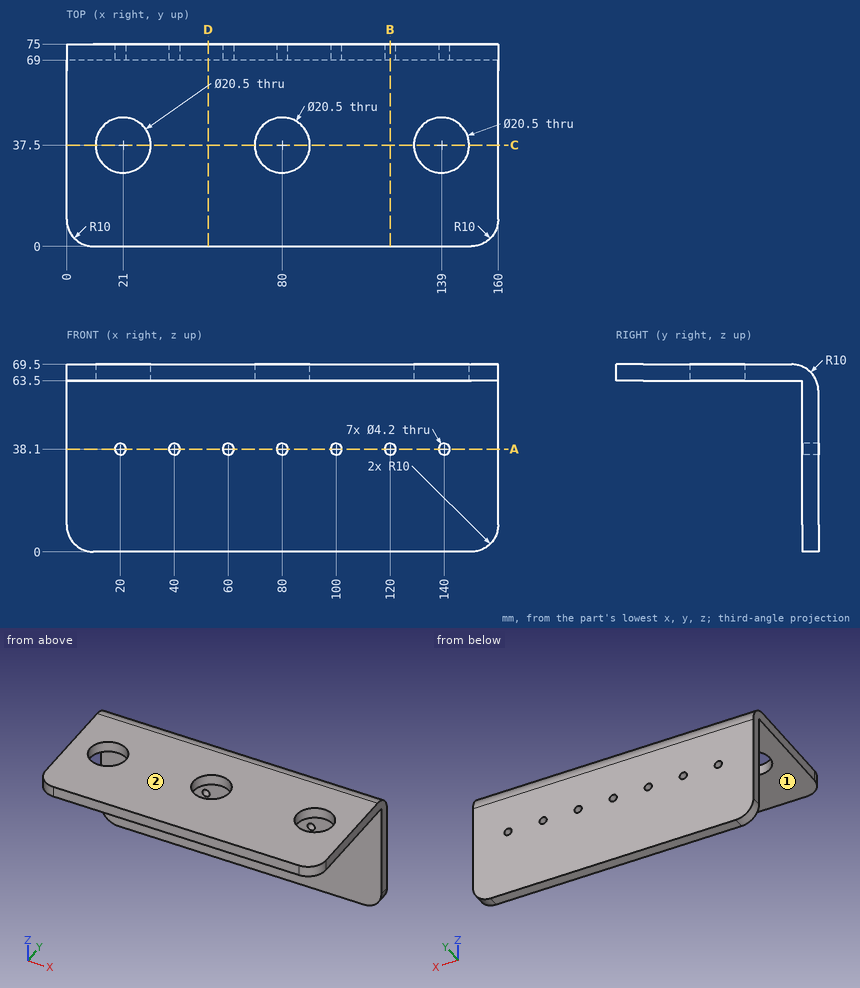
Part print with two shaded views. Sizes in mm from the minimum x, y, z corner. A direction names the side the tool comes from. Round coordinates to 2 decimals unless told otherwise and drop trailing zeros. Order: outer loops, then holes, each group sorted by start corner. A loop starts at its lowest first (then second) coordinate and runs counter-clockwise, first axis right, second up. Notation, with made-up numbers: (67.5, 42) - (104.5, 42) arc R32 cw to (104.5, 73) - close; hole circle Ø4 at (22.5, 56). An arc over 180 degrees is marked (long way). Answer in a Markdown table with one row per item. Add a question column.
(1) Drop flat-ended pins along their axis: pin 1 Ø3.5 at (x, z) = (100, 38.1) entering from +Y; pin 2 Ø12 at (x, z) = (106.5, 7.5) entering from -Y; pin 3 Ø23.5 at (x, y) = (21, 37.5) entering from -Z. Give the stop position or say it passes through.
(2) 3-axis set-ups, long thin cutter, end or side, ignore diameter. For the marked faces 1 and 2: which of +Z, -Z, +X, -X, +Y, -Y reach the whole face in a straight line?
(3) Band-saw the part on C-C on y = 37.5. List the corners of the cut face in (x, z), and give its area (3 significant figures).
(4) Band-saw the part on A-A on z = 38.1. Count the separate pieces of the cut face and the enclosed holes in it, and give its area (3 significant figures).
(5) Band-saw the part on D-D on x = 52.5. List the corners of the cut face in (y, z).
(6) Band-saw the part on B-B on x = 120. List the corners of the cut face in (y, z), and give its area (3 significant figures).
(7) Probe L1, parallel to X at y = 37, z = 67; L2, parallel to Y at x = 109.5, z = 54; L3, parallel to Z at x = 126.5, y = 24. List the from-to ranges inside material, lowest first. Write a range as [from, to].
Data:
| question | item | result |
|---|---|---|
| 1 | pin 1 | passes through |
| 1 | pin 2 | stops at y = 69 |
| 1 | pin 3 | stops at z = 63.5 |
| 2 | face 1 | -Z, +X, -X, -Y |
| 2 | face 2 | +Z, +X, -X, +Y, -Y |
| 3 | outline | (0, 63.5) - (10.75, 63.5) - (10.75, 69.5) - (0, 69.5) - close; (31.25, 63.5) - (69.75, 63.5) - (69.75, 69.5) - (31.25, 69.5) - close; (90.25, 63.5) - (128.75, 63.5) - (128.75, 69.5) - (90.25, 69.5) - close; (149.25, 63.5) - (160, 63.5) - (160, 69.5) - (149.25, 69.5) - close |
| 3 | area | 591 mm^2 |
| 4 | separate pieces | 8 |
| 4 | enclosed holes | 0 |
| 4 | area | 784 mm^2 |
| 5 | outline | (0, 63.5) - (69, 63.5) - (69, 0) - (75, 0) - (75, 59.5) arc R10 ccw to (65, 69.5) - (0, 69.5) - close |
| 6 | outline | (0, 63.5) - (69, 63.5) - (69, 40.2) - (75, 40.2) - (75, 59.5) arc R10 ccw to (65, 69.5) - (0, 69.5) - close; (69, 0) - (75, 0) - (75, 36) - (69, 36) - close |
| 6 | area | 784 mm^2 |
| 7 | L1 | x = [0, 10.76], [31.24, 69.76], [90.24, 128.76], [149.24, 160] |
| 7 | L2 | y = [69, 75] |
| 7 | L3 | z = [63.5, 69.5] |
